Can you work these out from the drawing? Everything is in mm from the part's minimum corner. A direction names the side the tool comes from. Round coordinates to 2 decimals unless told otherwise and drop trailing zeros. Loops run counter-clockwise (first coordinate to the right, second up) from the corner with the lowest first, then second, coordinate; pieces in that order, holes last. Notation, with made-up numbers: M 1,66.5 L 6,66.5 A10 cw 6,73.5 Z; hole C 2,60.5 d2. An arc over 180 degrees is marked long. One line per question, with ' | ' between items. Start each with the question number.
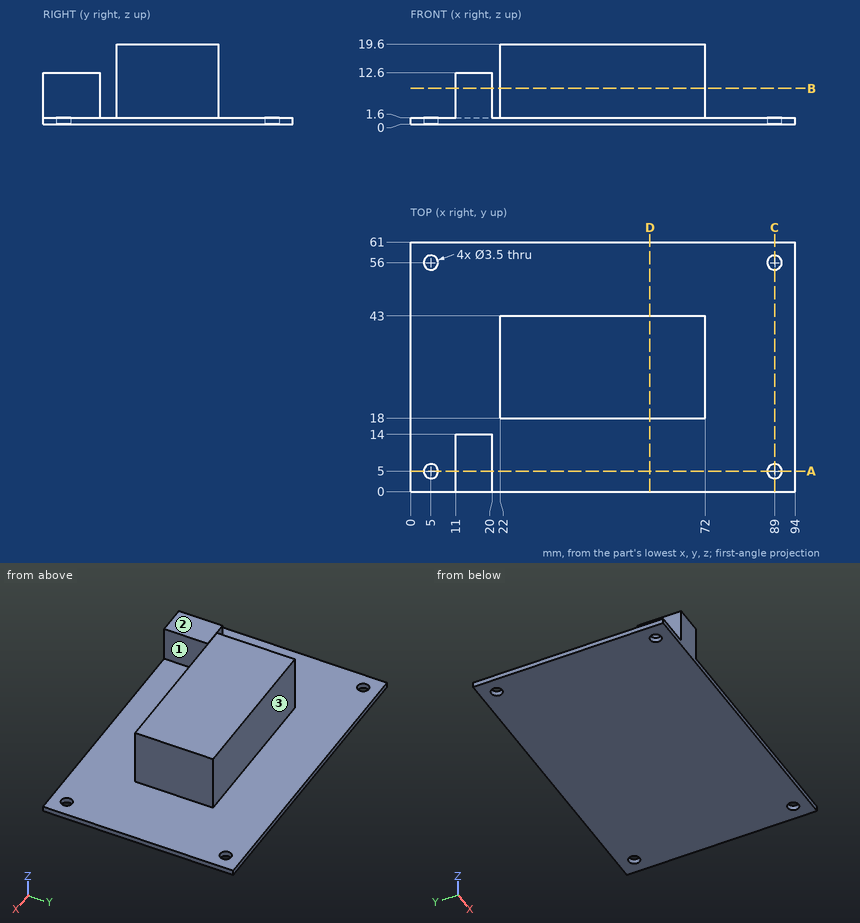
1) Imagine slicing it at C-C (x = 89). Write out the boundary of the cut face in (y, z), then the cut area to 3 significant figures.
2) Imagine slicing it at D-D (x = 58.5). Write out the boundary of the cut face in (y, z), then the cut area to 3 significant figures.
3) For the marked faces 1, 2 and 3, which set-ups out of +Z, -Z, +X, -X, +Y, -Y let a thin tool reach every point of the face, with its end or its side?
4) Imagine slicing it at B-B (z = 8.75). Write out the boundary of the cut face in (x, y), then the cut area to 3 significant figures.
5) I'm going to push flat-ended pins straight in: pin 1 Ø4 at (x, y) = (34, 22) entering from -Z; pin 2 Ø5.5 at (y, z) = (10, 10) entering from +X; pin 3 Ø3 at (y, z) = (23.5, 17.5) entering from +X; pin 4 Ø5 at (x, y) = (84.5, 18.5) entering from +Z. Where does each tip first touch, or does it pass through?
6) Please list where these lines run through material, in increasing order: L1, parallel to Y at x = 89, z = 0.55; L2, parallel to X at y = 23, z = 11.75; L3, parallel to Z at x = 18.5, y = 31. Write a range as from..to.
7) Imagine slicing it at A-A (y = 5). Write out the boundary of the cut face in (x, z).
Results are:
1) outline: M 0,0 L 3.25,0 L 3.25,1.6 L 0,1.6 Z; M 6.75,0 L 54.25,0 L 54.25,1.6 L 6.75,1.6 Z; M 57.75,0 L 61,0 L 61,1.6 L 57.75,1.6 Z | area: 86.4 mm²
2) outline: M 0,0 L 61,0 L 61,1.6 L 43,1.6 L 43,19.6 L 18,19.6 L 18,1.6 L 0,1.6 Z | area: 548 mm²
3) face 1: +Z, +X, +Y, -Y | face 2: +Z, +X, -X, +Y, -Y | face 3: +Z, +X, -X, +Y
4) outline: M 11,0 L 20,0 L 20,14 L 11,14 Z; M 22,18 L 72,18 L 72,43 L 22,43 Z | area: 1,380 mm²
5) pin 1: z = 0 | pin 2: x = 20 | pin 3: x = 72 | pin 4: z = 1.6
6) L1: 0..3.25, 6.75..54.25, 57.75..61 | L2: 22..72 | L3: 0..1.6
7) outline: M 0,0 L 3.25,0 L 3.25,1.6 L 0,1.6 Z; M 6.75,0 L 87.25,0 L 87.25,1.6 L 20,1.6 L 20,12.6 L 11,12.6 L 11,1.6 L 6.75,1.6 Z; M 90.75,0 L 94,0 L 94,1.6 L 90.75,1.6 Z
